from build123d import *

# Parameters (mm, degrees)
BOX001_W     = 480
BOX001_H     = 210
BOX001_DEPTH = 320
BOX_W        = 500
BOX_H        = 230
BOX_DEPTH    = 300
FILLET004_R  = 8


with BuildPart() as cube001:
    # Box001 → Box001 (new body)
    with BuildSketch(Plane(origin=(10, 10, 10), x_dir=(1, 0, 0), z_dir=(0, 0, 1))):
        with Locations((240, 105)):
            Rectangle(BOX001_W, BOX001_H)
    extrude(amount=BOX001_DEPTH)


with BuildPart() as solar_box:
    # Box → Box (new body)
    with BuildSketch(Plane.XY):
        with Locations((250, 115)):
            Rectangle(BOX_W, BOX_H)
    extrude(amount=BOX_DEPTH)

    # Cut: cut Cube001
    add(cube001.part, mode=Mode.SUBTRACT)

    # Fillet004
    fillet004_edges = [solar_box.edges().sort_by_distance(p)[0] for p in [
        (0, 0, 150),
        (0, 115, 300),
        (0, 230, 150),
        (0, 115, 0),
        (250, 0, 0),
        (500, 0, 150),
        (250, 0, 300),
        (250, 230, 300),
        (500, 115, 300),
        (250, 230, 0),
        (500, 230, 150),
        (500, 115, 0),
    ]]
    fillet(fillet004_edges, radius=FILLET004_R)


solid = solar_box.part
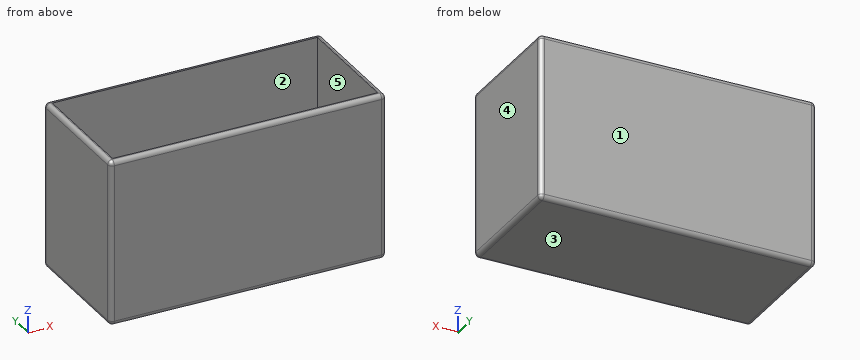
For this review, take the finished solid that the model builds, in its own axes (mm). Face numbers are marked on the shaded views. A direction names the side the tool comes from. Round coordinates to 2 decimals unless told otherwise and drop trailing zeros. Order: outer loops, then holes, each group sorted by start corner. A loop starts at its lowest first (then second) coordinate and runs counter-clockwise, first axis right, second up. Notation, with made-up numbers: M 29,-15.75 L 58,-15.75 A28 cw 58,23.25 Z; hole C 52.5,76.25 d5. An arc over 180 degrees is marked long. Use a Markdown table: item, result. Add a question column.
Item 1: Tool access review of the marked faces 4 and 5: name each direction out of +Z, -Z, +X, -X, +Y, -Y from which nothing blocks a thin tool from reaching the whole face with its end or side.
Item 2: Insertion check: pin 1 (2 mm diameter, centred on x = 354, y = 67, fed in from +Z). The pin has a flat end and moves straight along its axis. Give the tip position at first contact, or say it passes through.
Item 3: Add section A-A, the plane z = 162. Give the boundary of the cut face in (x, y).
Item 4: Mouldability with a two-part tool opening along Y and no side actions: class the marked faces 1, 2 and 3 as released by +Y, released by -Y, zero draft, split by the parting line, or undercut.
Item 5: Add section B-B, the plane x = 121.5. Give the boundary of the cut face in (y, z), then the cut area to 3 significant figures.
Item 6: Add section C-C, the plane y = 105. Give the boundary of the cut face in (x, z), then the cut area to 3 significant figures.
Item 7: To check wall thickness, follow line 1 along X through (y, z) = (35, 141.5); line 2 along Y through (x, z) = (44, 181.5); line 3 along Z through (x, y) = (464.5, 152). State the ranges of each line that lie inside material, in increasing order.
Geometry results:
| question | item | result |
|---|---|---|
| 1 | face 4 | +Z, -Z, +X, +Y, -Y |
| 1 | face 5 | +Z |
| 2 | pin 1 | stops at z = 10 |
| 3 | outline | M 0,8 A8 ccw 8,0 L 492,0 A8 ccw 500,8 L 500,222 A8 ccw 492,230 L 8,230 A8 ccw 0,222 Z; hole M 10,10 L 490,10 L 490,220 L 10,220 Z |
| 4 | face 1 | released by +Y |
| 4 | face 2 | undercut |
| 4 | face 3 | zero draft |
| 5 | outline | M 0,8 A8 ccw 8,0 L 222,0 A8 ccw 230,8 L 230,292 A8 ccw 222,300 L 220,300 L 220,10 L 10,10 L 10,300 L 8,300 A8 ccw 0,292 Z |
| 5 | area | 8,050 mm² |
| 6 | outline | M 0,8 A8 ccw 8,0 L 492,0 A8 ccw 500,8 L 500,292 A8 ccw 492,300 L 490,300 L 490,10 L 10,10 L 10,300 L 8,300 A8 ccw 0,292 Z |
| 6 | area | 10,700 mm² |
| 7 | line 1 | x = 0 to 10, 490 to 500 |
| 7 | line 2 | y = 0 to 10, 220 to 230 |
| 7 | line 3 | z = 0 to 10 |
